Drawing for the job (mm, zero at the part's lowest x, y, z). Give positions to 0.01 mm unless a question says otherwise; leave off trailing zeros. Order: outer loops, then holes, each group sorted by start corner. A loop starts at its lowest first (then second) coordinate and runs counter-clockwise, first axis right, second up. Notation, with made-up numbers: (40.5, 18) - (64.5, 18) arc R19 cw to (64.5, 38) - close; hole circle Ø11 at (81, 29). An arc over 180 degrees is marked (long way). Use a Markdown table: item, result. Add a question column.
(1) Wall check: line 1 (Z direction, x = 4.75, y = 1.95) (1 decimal); line 2 (Z direction, x = 3.5, y = 1.3) (1 decimal); line 3 (X direction, y = 1.7, z = 3.75). Give the ranges that are in metal, low to high.
(2) Mould opens along X. For the marked faces 1, 2 and 3 say: +X half, -X half, draft (parallel to the pull), parting line (faces both ways), or undercut.
(3) Slice it at A-A (y = 2.2). Write the cut outline in (x, z) (1 decimal).
(4) Flat gauge pin, fed straight in: pin 1 (1 mm diameter, centred on x = 1, y = 1, fed in from -Z). Where does the tip first touch, or does it go through?
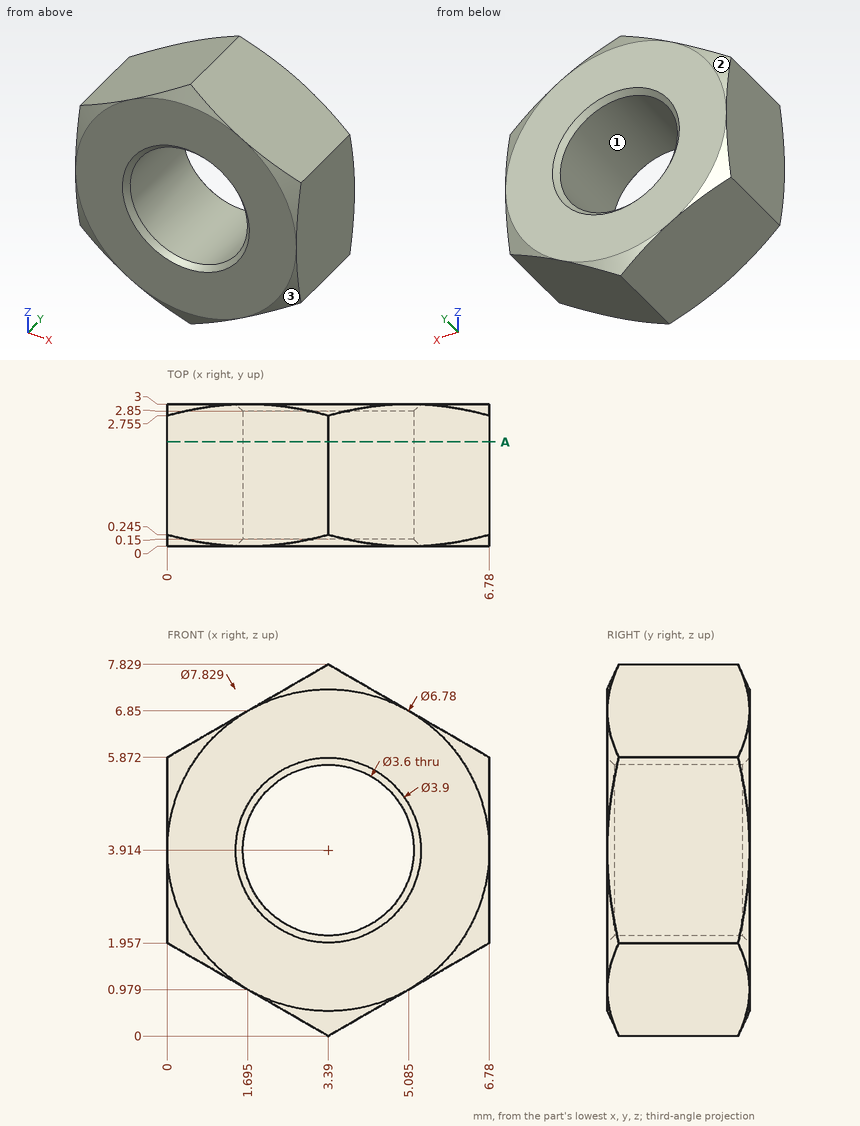
Solution:
| question | item | result |
|---|---|---|
| 1 | line 1 | 0.8 to 2.7, 5.1 to 7 |
| 1 | line 2 | 0.1 to 2.1, 5.7 to 7.8 |
| 1 | line 3 | 0 to 1.6, 5.18 to 6.78 |
| 2 | face 1 | undercut |
| 2 | face 2 | -X half |
| 2 | face 3 | +X half |
| 3 | outline | (0, 2) - (3.4, 0) - (6.8, 2) - (6.8, 5.9) - (3.4, 7.8) - (0, 5.9) - close; hole circle Ø3.6 at (3.4, 3.9) |
| 4 | pin 1 | z = 1.09 |
